Autodesk Inventor part; units mm, degrees
ref_plane "Work Plane1" through (7.95, 0, 0) normal (1, 0, 0) x (0, 1, 0)
ref_plane "XZ Plane" through (0, 0, 0) normal (0, 1, 0) x (-1, 0, 0)
ref_plane "XY Plane" through (0, 0, 0) normal (0, 0, 1) x (1, 0, 0)
sketch "Sketch1" plane through (0, 0, 0) normal (0, 1, 0) x (-1, 0, 0)
  circle A0 centre (0, 0) radius 4
  circle A1 centre (0, 0) radius 7.95
  dimension "d0" = 8
  dimension "d1" = 15.9
extrude "Extrusion1" add sketch "Sketch1" along normal blind 8
ref_plane "Work Plane1" through (7.95, 0, 0) normal (1, 0, 0) x (0, 1, 0)
sketch "Sketch2" plane through (7.95, 0, 0) normal (1, 0, 0) x (0, 1, 0)
  circle A0 centre (4, 0) radius 1.5
  line L0 (0, -7.95) -> (0, 7.95)
  line L1 (8, -7.95) -> (8, 7.95)
  point P0 (0, 0)
  dimension "d4" = 3
  dimension "d5" = 8
  dimension "d6" = 4
extrude "Extrusion2" cut sketch "Sketch2" against normal up to surface
thread "Thread1"
chamfer "Chamfer1" distance 0.5 angle 45 7 edges at (7.95, 8, 0) (4, 8, 0) (7.95, 0, 0) (4, 0, 0) (4, 2.5, -0.0003) (7.8072, 3.9998, -1.5) (7.8072, 4.0001, 1.5)
properties part number "stelring - 8mm" material "Stainless Steel"
The listing builds one solid part. Answer for the finished solid, in the listing's coordinates (mm). A direction names the side the tool comes from. Give positions to 0.01 mm unless a question says otherwise; leave off trailing zeros. Write each loop counter-clockwise with the first axis right and the second up, starting at its lowest first coordinate (ties: lowest second). Pieces come first, ordered by that corner, then holes. Notation, with made-up numbers: (-1, 45.25) - (51, 45.25) arc R17 ccw to (51, 50.25) - close; hole circle Ø1 at (5.25, 29). An arc over 180 degrees is marked (long way). Use a Markdown table: item, result.
1. Section B-B on y = 1.25 is taken. Write down the section's boundary in (x, z), plus the area to 3 significant figures.
Values follow:
| item | result |
|---|---|
| outline | circle Ø15.9 at (0, 0); hole circle Ø8 at (0, 0) |
| area | 148 mm² |
2. Section C-C on z = 0.5 is taken. Count the separate pieces of the cut face and the enclosed holes in it, plus the area to 3 significant figures.
Values follow:
| item | result |
|---|---|
| separate pieces | 3 |
| enclosed holes | 0 |
| area | 50.7 mm² |
3. Section A-A on x = 0 is taken. Write down the section's boundary in (y, z), plus the area to 3 significant figures.
Values follow:
| item | result |
|---|---|
| outline | (0, -7.45) - (0.5, -7.95) - (7.5, -7.95) - (8, -7.45) - (8, -4.5) - (7.5, -4) - (0.5, -4) - (0, -4.5) - close; (0, 4.5) - (0.5, 4) - (7.5, 4) - (8, 4.5) - (8, 7.45) - (7.5, 7.95) - (0.5, 7.95) - (0, 7.45) - close |
| area | 62.2 mm² |
4. Each of these flat-tipped pins is pushed along its axis until it touches: P1, Ø6, axis at x = 2, z = 0.5, coming from the +Y side; P2, Ø2, axis at x = 5, y = 5, coming from the -Z side. Where does it stop, or does it pass through?
Values follow:
| item | result |
|---|---|
| P1 | stops at y = 8 |
| P2 | stops at z = -6.87 |
5. For a pull along Z with two mould halves and no side action, classify faces 1 (the flat face through (0, 0, -5)), 2 (the cylindrical face through (-7.583, 3.951, -2.388)), 3 (the cylindrical face through (-3.695, 3.951, 1.532)) as released by +Z, released by -Z, zero draft, split by the parting line, or undercut.
Values follow:
| item | result |
|---|---|
| face 1 | zero draft |
| face 2 | split by the parting line |
| face 3 | undercut |
6. Find the intervals of material crossed by probe 1 along Z at (x, y) = (0, 4); probe 2 along X at (y, z) = (5, 0); probe 3 along X at (y, z) = (1.25, 3.25), in increasing order. Write a range as from..to.
Values follow:
| item | result |
|---|---|
| probe 1 | z = -7.95..-4, 4..7.95 |
| probe 2 | x = -7.95..-4 |
| probe 3 | x = -7.26..-2.33, 2.33..7.26 |
7. A tool of negligible diameter and unlimited length cuts with its end or side. For faces 4 (the flat face through (0, 8, -5)), 5 (the cylindrical face through (5.85, 2.5, 0.07)), from which of +Z, -Z, +X, -X, +Y, -Y can it reach the whole face along a straight path? Write none if from no direction.
Values follow:
| item | result |
|---|---|
| face 4 | +Z, -Z, +X, -X, +Y |
| face 5 | +X |
